Drawing for the job (mm, zero at the part's lowest x, y, z). Round coordinates to 2 decimals unless told otherwise and drop trailing zeros. Write each loop counter-clockwise with the first axis right and the second up, starting at its lowest first coordinate (ties: lowest second). Pieces come first, ordered by that corner, then holes. Notation, with made-up numbers: (-19, 11) -> (3, 11) arc R17 ccw to (3, 36) -> close; hole circle Ø1 at (67, 13.25). An arc over 180 degrees is marked (long way). Answer in a Markdown table with one row per item. Add a question column.
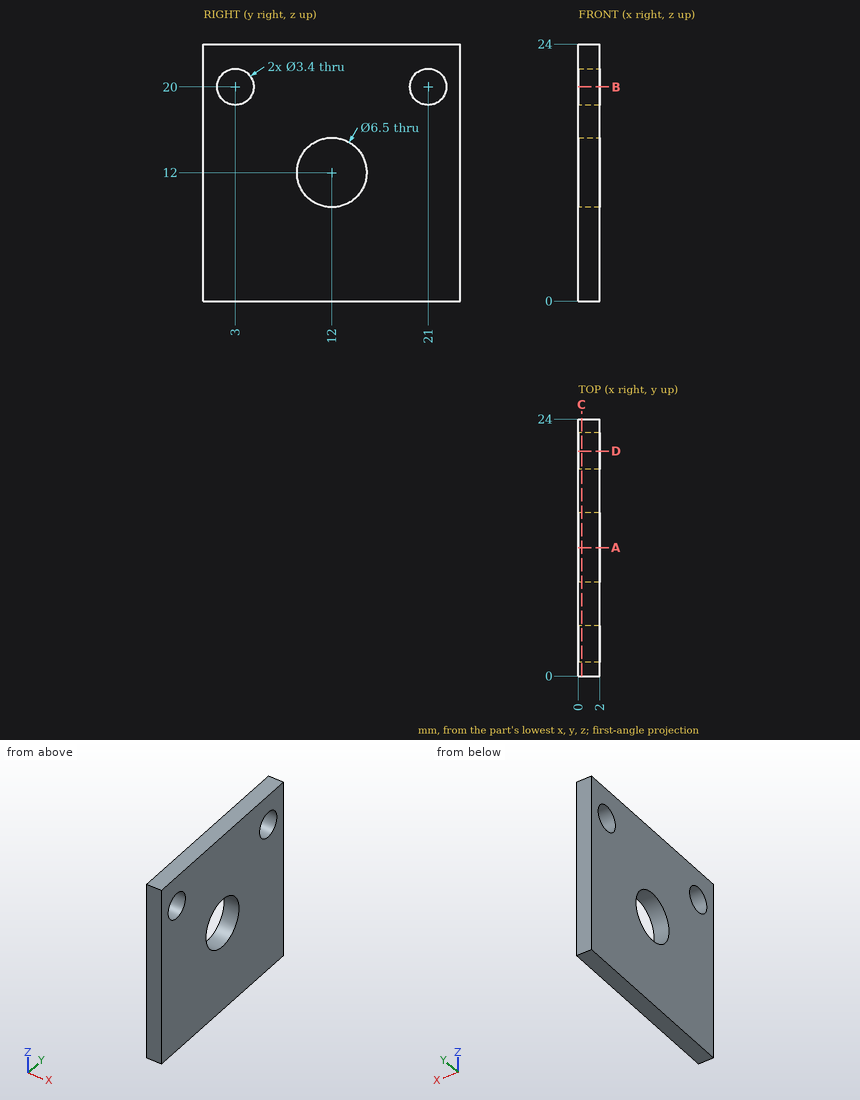
(1) Drop a flat-ended pin along its axis: P1, Ø6, axis at y = 12, z = 12, coming from the -X side. Give the stop position or say it passes through.
(2) Saw through at C-C (x = 0.3). List the corners of the cut face in (y, z).
(3) Probe line 1 along Y through (x, z) = (1.4, 20); line 2 along Y through (x, z) = (0.3, 20.5); line 3 along Y through (x, z) = (1.6, 12). List the from-to ranges inside material, lowest first.
(4) Saw through at D-D (y = 21). List the corners of the cut face in (x, z).
(5) Saw through at A-A (y = 12). List the corners of the cut face in (x, z).
(6) Saw through at B-B (z = 20). List the corners of the cut face in (x, y).
Answer sheet:
| question | item | result |
|---|---|---|
| 1 | P1 | passes through |
| 2 | outline | (0, 0) -> (24, 0) -> (24, 24) -> (0, 24) -> close; hole circle Ø3.4 at (3, 20); hole circle Ø6.5 at (12, 12); hole circle Ø3.4 at (21, 20) |
| 3 | line 1 | y = 0 to 1.3, 4.7 to 19.3, 22.7 to 24 |
| 3 | line 2 | y = 0 to 1.38, 4.62 to 19.38, 22.62 to 24 |
| 3 | line 3 | y = 0 to 8.75, 15.25 to 24 |
| 4 | outline | (0, 0) -> (2, 0) -> (2, 18.3) -> (0, 18.3) -> close; (0, 21.7) -> (2, 21.7) -> (2, 24) -> (0, 24) -> close |
| 5 | outline | (0, 0) -> (2, 0) -> (2, 8.75) -> (0, 8.75) -> close; (0, 15.25) -> (2, 15.25) -> (2, 24) -> (0, 24) -> close |
| 6 | outline | (0, 0) -> (2, 0) -> (2, 1.3) -> (0, 1.3) -> close; (0, 4.7) -> (2, 4.7) -> (2, 19.3) -> (0, 19.3) -> close; (0, 22.7) -> (2, 22.7) -> (2, 24) -> (0, 24) -> close |
